Design review of the part built by this model. Coordinates are the model's own, in mm. A direction names the side the tool comes from. Give positions to 0.01 mm unless a question says otherwise; leave off trailing zeros. Loops run counter-clockwise (first coordinate to the right, second up) from the corner with the lowest first, then second, coordinate; pieces in that order, holes last. Notation, with made-up numbers: M 26.5,64 L 31.5,64 A31 ccw 31.5,97 Z; hole C -32,44.25 d10. An arc over 180 degrees is marked long. Use a Markdown table: item, result. Add a question column.
(1) For faces 4 (the face through (14.5, 1, 0)), 5 (the face through (4, 4, 0)), list the 3-axis set-ups (+Z, -Z, +X, -X, +Y, -Y) from which the entire face can be reached by the end or side of a thin tool; tool diameter is ignored.
(2) For probe 1 along X at (y, z) = (5.15, -6); probe 2 along X at (y, z) = (2.1, -7); probe 3 along Z at (x, y) = (6.5, 4), list the stretches that pass through material, from the lowest coordinate up.
(3) Add section C-C, the plane y = 3.45. State how many separate pieces and enclosed holes the cut face has, then the cut area to 3 significant figures.
(4) Add section A-A, the plane z = -6. Give the boundary of the cut face in (x, y), then the cut area to 3 significant figures.
(5) Draft analysis for pull direction X (two halves, no side actions). For faces 1 (the face through (-0.3, 4.5, -4.4)), 2 (the face through (20, 3, 0)), 3 (the face through (-5, 0, -4)), state which applies: pulls with the +X half, pulls with the -X half, needs draft (parallel to the pull), parting line crosses it, or undercut.
(6) Add section B-B, the plane x = -8.5. Give the boundary of the cut face in (y, z).
(7) Insertion check: pin 1 Ø3.5 at (x, z) = (0, 0) entering from +Y; pin 2 Ø3 at (x, z) = (-13, -3.5) entering from -Y; pin 3 Ø1.5 at (x, z) = (-1.5, -3) entering from -Y. Each pin has a flat end and moves straight along its axis. Give the tip position at first contact, or say it passes through.
(8) Add section D-D, the plane x = 11.5. Give the boundary of the cut face in (y, z).
```python
from build123d import *

# Parameters (mm, degrees)
SKETCH1_W           = 40
SKETCH1_H           = 30
BOSS_EXTRUDE1_DEPTH = 3
SKETCH2_W           = 40
SKETCH2_H           = 30
SKETCH2_R           = 2
SKETCH2_R_2         = 0.5
BOSS_EXTRUDE2_DEPTH = 3


with BuildPart() as part:
    # Sketch1 → Boss-Extrude1 (new body)
    with BuildSketch(Plane(origin=(0, 0, 0), x_dir=(1, 0, 0), z_dir=(0, 1, 0))):
        Rectangle(SKETCH1_W, SKETCH1_H)
        Polygon((-2.55, -2.55), (-2.55, -7.85), (2.55, -7.85), (2.55, -2.55), (14.5, -2.55), (14.5, 2.55), (2.55, 2.55), (2.55, 7.85), (-2.55, 7.85), (-2.55, 2.55), (-14.5, 2.55), (-14.5, -2.55), align=None, mode=Mode.SUBTRACT)
    extrude(amount=BOSS_EXTRUDE1_DEPTH)

    # Sketch2 → Boss-Extrude2 (add)
    with BuildSketch(Plane(origin=(0, 3, 0), x_dir=(1, 0, 0), z_dir=(0, 1, 0))):
        Rectangle(SKETCH2_W, SKETCH2_H)
        with Locations(Location((0, 0, 0), (0, 0, 270))):
            Circle(SKETCH2_R, mode=Mode.SUBTRACT)
        with Locations(Location((-4.5, 0, 0), (0, 0, 270))):
            Circle(SKETCH2_R_2, mode=Mode.SUBTRACT)
        with Locations(Location((-6.5, 0, 0), (0, 0, 270))):
            Circle(SKETCH2_R_2, mode=Mode.SUBTRACT)
        with Locations(Location((-8.5, 0, 0), (0, 0, 270))):
            Circle(SKETCH2_R_2, mode=Mode.SUBTRACT)
        with Locations(Location((-10.5, 0, 0), (0, 0, 270))):
            Circle(SKETCH2_R_2, mode=Mode.SUBTRACT)
        with Locations(Location((-12.5, 0, 0), (0, 0, 270))):
            Circle(SKETCH2_R_2, mode=Mode.SUBTRACT)
        with Locations(Location((0, 4, 0), (0, 0, 270))):
            Circle(SKETCH2_R_2, mode=Mode.SUBTRACT)
        with Locations(Location((0, 6, 0), (0, 0, 270))):
            Circle(SKETCH2_R_2, mode=Mode.SUBTRACT)
        with Locations(Location((12.5, 0, 0), (0, 0, 90))):
            Circle(SKETCH2_R_2, mode=Mode.SUBTRACT)
        with Locations(Location((10.5, 0, 0), (0, 0, 90))):
            Circle(SKETCH2_R_2, mode=Mode.SUBTRACT)
        with Locations(Location((8.5, 0, 0), (0, 0, 90))):
            Circle(SKETCH2_R_2, mode=Mode.SUBTRACT)
        with Locations(Location((6.5, 0, 0), (0, 0, 90))):
            Circle(SKETCH2_R_2, mode=Mode.SUBTRACT)
        with Locations(Location((4.5, 0, 0), (0, 0, 90))):
            Circle(SKETCH2_R_2, mode=Mode.SUBTRACT)
        with Locations(Location((0, -4, 0), (0, 0, 90))):
            Circle(SKETCH2_R_2, mode=Mode.SUBTRACT)
        with Locations(Location((0, -6, 0), (0, 0, 90))):
            Circle(SKETCH2_R_2, mode=Mode.SUBTRACT)
    extrude(amount=BOSS_EXTRUDE2_DEPTH)


solid = part.part
```
Established:
| question | item | result |
|---|---|---|
| 1 | face 4 | -Y |
| 1 | face 5 | +Y, -Y |
| 2 | probe 1 | -20 to -0.5, 0.5 to 20 |
| 2 | probe 2 | -20 to -2.55, 2.55 to 20 |
| 2 | probe 3 | -15 to -0.5, 0.5 to 15 |
| 3 | separate pieces | 1 |
| 3 | enclosed holes | 15 |
| 3 | area | 1,180 mm^2 |
| 4 | outline | M -20,0 L -2.55,0 L -2.55,3 L -0.5,3 L -0.5,6 L -20,6 Z; M 0.5,3 L 2.55,3 L 2.55,0 L 20,0 L 20,6 L 0.5,6 Z |
| 4 | area | 222 mm^2 |
| 5 | face 1 | undercut |
| 5 | face 2 | pulls with the +X half |
| 5 | face 3 | needs draft |
| 6 | outline | M 0,-15 L 6,-15 L 6,-0.5 L 3,-0.5 L 3,-2.55 L 0,-2.55 Z; M 0,2.55 L 3,2.55 L 3,0.5 L 6,0.5 L 6,15 L 0,15 Z |
| 7 | pin 1 | through |
| 7 | pin 2 | y = 0 |
| 7 | pin 3 | y = 3 |
| 8 | outline | M 0,-15 L 6,-15 L 6,15 L 0,15 L 0,2.55 L 3,2.55 L 3,-2.55 L 0,-2.55 Z |
